Input: dimensioned drawing with shaded views. Units: mm. Origin: part minimum x, y, z. A direction names the side the tool comes from. Coordinates: 2 decimals unless noted, no trailing zeros. Loops run counter-clockwise (first coordinate to the right, second up) from the corner with the lowest first, then second, coordinate; pieces in that order, holes last.
(1) Contact query for flat-ended pins moving along their axis: P1, Ø3, axis at y = 29.5, z = 36, coming from the -X side (1 decimal); P2, Ø2, axis at x = 67.5, z = 66, coming from the +Y side (1 decimal); P3, Ø8, axis at x = 43.06, z = 6.3, coming from the -Y side. Output: stop coordinate, or through.
(2) Section B-B, the plane x = 14. Return loops of the section in (y, z) (1 decimal).
(3) Set-up query: the marked faces 1 and 2. Return all of +Z, -Z, +X, -X, +Y, -Y with unobstructed straight access to the full face (end or side cutting, diameter ignored); none if empty.
(4) Section C-C, the plane z = 88.9. Return loops of the section in (x, y) (1 decimal).
(5) Section D-D, the plane y = 35.5. Return loops of the section in (x, z) (1 decimal).
(6) Section A-A, the plane z = 63.5. Return loops of the section in (x, y) (1 decimal).
(7) Line query: L1, parallel to X at y = 12.5, z = 84 (1 decimal); L2, parallel to Y at x = 75, z = 38; L3, parallel to Y at x = 23, z = 36 (1 decimal). Output: solid intervals per line, ascending.
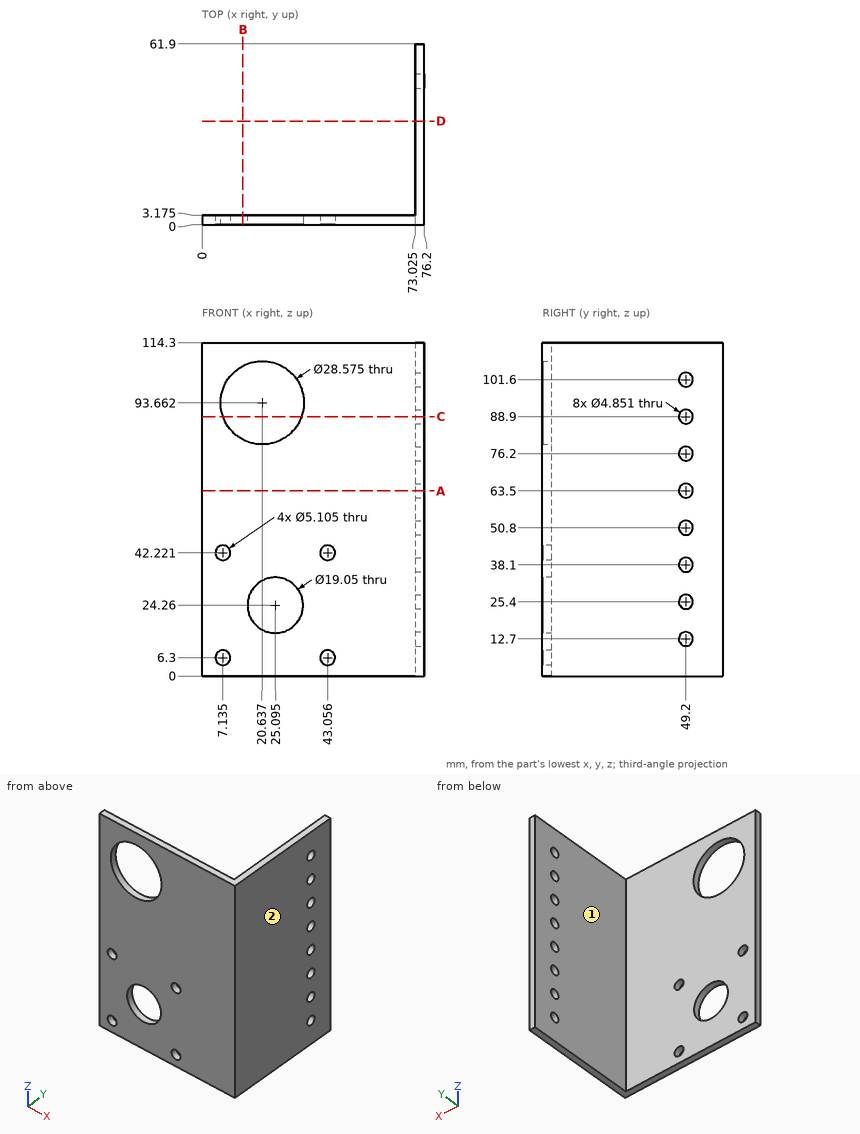
Report:
1. P1: stops at x = 73
1. P2: stops at y = 3.2
1. P3: stops at y = 0
2. outline: (0, 0) - (3.2, 0) - (3.2, 81) - (0, 81) - close; (0, 106.3) - (3.2, 106.3) - (3.2, 114.3) - (0, 114.3) - close
3. face 1: +Z, -Z, -X, +Y
3. face 2: +Z, -Z, +X, +Y, -Y
4. outline: (0, 0) - (7.2, 0) - (7.2, 3.2) - (0, 3.2) - close; (34.1, 0) - (76.2, 0) - (76.2, 46.8) - (73, 46.8) - (73, 3.2) - (34.1, 3.2) - close; (73, 51.6) - (76.2, 51.6) - (76.2, 61.9) - (73, 61.9) - close
5. outline: (73, 0) - (76.2, 0) - (76.2, 114.3) - (73, 114.3) - close
6. outline: (0, 0) - (76.2, 0) - (76.2, 46.8) - (73, 46.8) - (73, 3.2) - (0, 3.2) - close; (73, 51.6) - (76.2, 51.6) - (76.2, 61.9) - (73, 61.9) - close
7. L1: x = 73 to 76.2
7. L2: y = 0 to 46.78, 51.62 to 61.9
7. L3: y = 0 to 3.2
